Design review of the part built by this model. Coordinates are the model's own, in mm. Face numbers are marked on the shaded views. A direction names the side the tool comes from. Give positions to 0.01 mm unless a question says otherwise; leave off trailing zeros. Order: outer loops, then holes, each group sorted by start corner. A loop starts at its lowest first (then second) coordinate and runs counter-clockwise, first axis right, second up. Notation, with made-up numbers: (-23, -12) -> (22, -12) arc R5 ccw to (22, -8) -> close; hole circle Ø6 at (46.5, 64). An arc over 180 degrees is marked (long way). One line per item, written item: value. Start each with the question number.
1) The part is to be moulded in two halves that separate along X. For the marked faces 3, 4, 5 and 6, say which applies: released by +X, released by -X, zero draft, split by the parting line, or undercut.
2) For pin 1 (5 mm diameter, centred on x = 9, z = 3.5, fed in from +Y), flat-tipped, find the tip position at first contact; note if it passes through.
3) Tool access review of the marked faces 1 and 2: name each direction out of +Z, -Z, +X, -X, +Y, -Y from which nothing blocks a thin tool from reaching the whole face with its end or side.
4) Consider section C-C (x = 31.75). State the section outline as (y, z) points, plus the area to 3 significant figures.
5) Wall thickness on line 1 along Y through (x, z) = (-31.75, 8.25); line 2 along X through (y, z) = (-19.05, 3.5); line 3 along X through (y, z) = (19.05, 3.75): over which ranges is each line inside the solid? List them lowest first. Write a range as from..to.
6) Consider section B-B (z = 4). State the section outline as (x, y) points.
7) Consider section A-A (y = -19.05). State the section outline as (x, z) points, plus the area to 3 significant figures.
8) Consider section D-D (y = 19.05). State the section outline as (x, z) points.
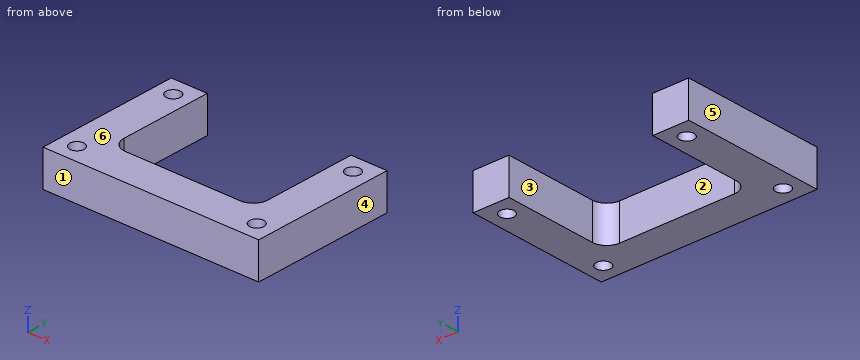
from build123d import *

# Parameters (mm, degrees)
BOSS_EXTRUDE1_DEPTH     = 12.7
SKETCH4_R               = 2.54
CUT_EXTRUDE3_DEPTH      = 13.7
CUT_EXTRUDE3_DEPTH_BACK = 1
FILLET1_R               = 5.08


with BuildPart() as part:
    # Sketch2 → Boss-Extrude1 (new body)
    with BuildSketch(Plane.XY):
        Polygon((-25.4, 25.4), (-25.4, -12.7), (25.4, -12.7), (25.4, 25.4), (38.1, 25.4), (38.1, -25.4), (-38.1, -25.4), (-38.1, 25.4), align=None)
    extrude(amount=BOSS_EXTRUDE1_DEPTH)

    # Sketch4 → Cut-Extrude3 (cut, two sides)
    with BuildSketch(Plane.XY) as cut_extrude3_sk:
        with Locations((-31.75, 19.05)):
            Circle(SKETCH4_R)
        with Locations((31.75, 19.05)):
            Circle(SKETCH4_R)
        with Locations((31.75, -19.05)):
            Circle(SKETCH4_R)
        with Locations((-31.75, -19.05)):
            Circle(SKETCH4_R)
    extrude(amount=CUT_EXTRUDE3_DEPTH, mode=Mode.SUBTRACT)
    extrude(cut_extrude3_sk.sketch, amount=-CUT_EXTRUDE3_DEPTH_BACK, mode=Mode.SUBTRACT)

    # Fillet1
    fillet1_edges = [part.edges().sort_by_distance(p)[0] for p in [
        (-25.4, -12.7, 6.35),
        (25.4, -12.7, 6.35),
    ]]
    fillet(fillet1_edges, radius=FILLET1_R)


solid = part.part
Checked values:
1. face 3: undercut
1. face 4: released by +X
1. face 5: released by -X
1. face 6: zero draft
2. pin 1: stops at y = -12.7
3. face 1: +Z, -Z, +X, -X, -Y
3. face 2: +Z, -Z, +Y
4. outline: (-25.4, 0) -> (-21.59, 0) -> (-21.59, 12.7) -> (-25.4, 12.7) -> close; (-16.51, 0) -> (16.51, 0) -> (16.51, 12.7) -> (-16.51, 12.7) -> close; (21.59, 0) -> (25.4, 0) -> (25.4, 12.7) -> (21.59, 12.7) -> close
4. area: 516 mm^2
5. line 1: y = -25.4..-21.59, -16.51..16.51, 21.59..25.4
5. line 2: x = -38.1..-34.29, -29.21..29.21, 34.29..38.1
5. line 3: x = -38.1..-34.29, -29.21..-25.4, 25.4..29.21, 34.29..38.1
6. outline: (-38.1, -25.4) -> (38.1, -25.4) -> (38.1, 25.4) -> (25.4, 25.4) -> (25.4, -7.62) arc R5.08 cw to (20.32, -12.7) -> (-20.32, -12.7) arc R5.08 cw to (-25.4, -7.62) -> (-25.4, 25.4) -> (-38.1, 25.4) -> close; hole circle Ø5.08 at (-31.75, -19.05); hole circle Ø5.08 at (-31.75, 19.05); hole circle Ø5.08 at (31.75, -19.05); hole circle Ø5.08 at (31.75, 19.05)
7. outline: (-38.1, 0) -> (-34.29, 0) -> (-34.29, 12.7) -> (-38.1, 12.7) -> close; (-29.21, 0) -> (29.21, 0) -> (29.21, 12.7) -> (-29.21, 12.7) -> close; (34.29, 0) -> (38.1, 0) -> (38.1, 12.7) -> (34.29, 12.7) -> close
7. area: 839 mm^2
8. outline: (-38.1, 0) -> (-34.29, 0) -> (-34.29, 12.7) -> (-38.1, 12.7) -> close; (-29.21, 0) -> (-25.4, 0) -> (-25.4, 12.7) -> (-29.21, 12.7) -> close; (25.4, 0) -> (29.21, 0) -> (29.21, 12.7) -> (25.4, 12.7) -> close; (34.29, 0) -> (38.1, 0) -> (38.1, 12.7) -> (34.29, 12.7) -> close
